```python
from build123d import *

# Parameters (mm, degrees)
BOSS_EXTRUDE2_DEPTH = 503
SHELL1_START        = -463
SHELL1_DEPTH        = 926
FILLET1_R           = 10
SKETCH8_W           = 131.571198008
SKETCH8_H           = 57.2
CUT_EXTRUDE5_DEPTH  = 1006
LPATTERN1_COUNT     = 5
LPATTERN1_PITCH     = 177.2
BOSS_EXTRUDE4_START = -350
SKETCH12_R          = 38
BOSS_EXTRUDE4_DEPTH = 50


# Read off the part's stored shape, not the designer's step: Shell1
with BuildPart() as part:
    # Sketch1 → Boss-Extrude2 (new, symmetric)
    with BuildSketch(Plane.XY):
        with BuildLine():
            ThreePointArc((-150, 150), (-106.066017178, 43.933982822), (0, 0))
            Line((0, 0), (758, 0))
            Line((758, 0), (758, -25))
            Line((758, -25), (777.984855583, -25))
            Line((777.984855583, -25), (794.363516125, 20))
            Line((794.363516125, 20), (356.523002694, 778.362014874))
            Line((356.523002694, 778.362014874), (50.523002694, 778.362014874))
            Line((50.523002694, 778.362014874), (-150, 300))
            Line((-150, 300), (-150, 150))
        make_face()
        Polygon((794.363516125, 20), (777.984855583, -25), (918, -25), align=None)
    extrude(amount=BOSS_EXTRUDE2_DEPTH, both=True)

    # Shell1 outline → Shell1 (cut)
    with BuildSketch(Plane.XY.offset(SHELL1_START)):
        with BuildLine():
            ThreePointArc((-110, 150), (-77.781745931, 72.218254069), (0, 40))
            Line((0, 40), (782.816510741, 40))
            Line((782.816510741, 40), (379.617013461, 738.362014874))
            Line((379.617013461, 738.362014874), (77.127737155, 738.362014874))
            Line((77.127737155, 738.362014874), (-110, 291.955367349))
            Line((-110, 291.955367349), (-110, 150))
        make_face()
    extrude(amount=SHELL1_DEPTH, mode=Mode.SUBTRACT)

    # Fillet1
    fillet1_edges = [part.edges().sort_by_distance(p)[0] for p in [
        (-77.781745931, 72.218254069, 463),
        (391.408255371, 40, -463),
        (-16.436131422, 515.158691112, 463),
        (-110, 220.977683675, 463),
        (391.408255371, 40, 463),
        (-77.781745931, 72.218254069, -463),
        (-110, 220.977683675, -463),
        (-16.436131422, 515.158691112, -463),
    ]]
    fillet(fillet1_edges, radius=FILLET1_R)

    # Sketch8 → Cut-Extrude5 (cut)
    with BuildSketch(Plane(origin=(99.350755487, 272.963957307, 0), x_dir=(0.9396926207859106, -0.3420201433256628, 0), z_dir=(0.34202014332566283, 0.9396926207859106, 0))):
        with Locations((805.402730461, 354.4)):
            Rectangle(SKETCH8_W, SKETCH8_H)
    cut_extrude5 = extrude(amount=-CUT_EXTRUDE5_DEPTH, mode=Mode.SUBTRACT)

    # LPattern1: Cut-Extrude5 ×5
    with Locations(*[(0, 0, i * LPATTERN1_PITCH) for i in range(1, LPATTERN1_COUNT)]):
        add(cut_extrude5, mode=Mode.SUBTRACT)

    # Sketch12 → Boss-Extrude4 (add)
    with BuildSketch(Plane.XY.offset(503).offset(BOSS_EXTRUDE4_START)):
        with BuildLine():
            Line((366.724091876, 760.693210118), (431.275772112, 872.5))
            ThreePointArc((431.275772112, 872.5), (431.275772112, 947.5), (366.323866828, 985))
            Line((366.323866828, 985), (-18.476997306, 985))
            ThreePointArc((-18.476997306, 985), (-71.510005895, 963.033008589), (-93.476997306, 910))
            Line((-93.476997306, 910), (-93.476997306, 434.839679698))
            Line((-93.476997306, 434.839679698), (50.523002694, 778.362014874))
            Line((50.523002694, 778.362014874), (356.523002694, 778.362014874))
            Line((356.523002694, 778.362014874), (366.724091876, 760.693210118))
        make_face()
        with Locations((-18.476997306, 910)):
            Circle(SKETCH12_R, mode=Mode.SUBTRACT)
        with Locations((366.323866828, 910)):
            Circle(SKETCH12_R, mode=Mode.SUBTRACT)
    boss_extrude4 = extrude(amount=BOSS_EXTRUDE4_DEPTH)

    # Mirror2: Boss-Extrude4 across plane
    add(boss_extrude4.mirror(Plane.XY))


solid = part.part
```
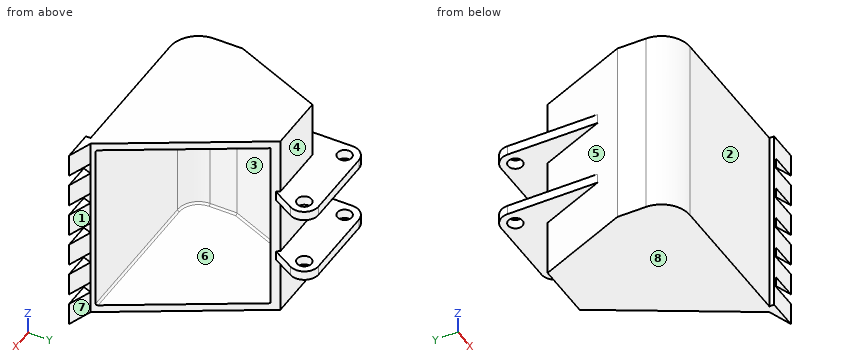
Model file for the job. Use its own axes, mm. Face numbers are marked on the shaded views. A direction names the side the tool comes from. Give positions to 0.01 mm unless a question says otherwise; leave off trailing zeros. Write each loop counter-clockwise with the first axis right and the second up, starting at its lowest first coordinate (ties: lowest second). Pieces come first, ordered by that corner, then holes. Notation, with made-up numbers: (12, 10) -> (18, 10) arc R20 cw to (18, 46) -> close; hole circle Ø3 at (32, -1). An arc over 180 degrees is marked (long way). Use CSV: the item, a comma, the result in double quotes. Start each with the question number.
1) Drill centre lines: L1, parallel to Z at x = 442.5, y = 555; L2, parallel to Y at x = 256, z = 350; L3, parallel to Y at x = 357, z = -198.5. Where is each one in solid material? Low to high.
2) Two-plate mould, pull along Y, no slides. Class the marked faces 6, 7 and 8: released by +Y, released by -Y, zero draft, split by the parting line, or undercut.
3) Cut at A-A on x = 128. List the corners of the cut face in (y, z), plus the area to 3 significant figures.
4) Pin check, flat tips, straight feed: P1, Ø1.5, axis at x = 266, z = -104.5, coming from the +Y side; P2, Ø1, axis at y = 751, z = 374.5, coming from the -X side; P3, Ø5, axis at x = -34.5, z = -109, coming from the -Y side. Stop position of each tip, or through.
5) Cut at B-B on z = 245. List the corners of the cut face in (x, y).
6) Cut at C-C on x = 619. List the corners of the cut face in (y, z), plus the area to 3 significant figures.
7) Tool access for the marked faces 1, 2, 3, 4 and 5: list every direction of +Z, -Z, +X, -X, +Y, -Y with a clear straight run to the whole face (end or side of a thin tool).
Final values:
1,L1,"z = -503 to -463, 463 to 503"
1,L2,"y = 0 to 40, 738.36 to 778.36"
1,L3,"y = 0 to 40, 738.36 to 873.16, 946.84 to 985"
2,face 6,"undercut"
2,face 7,"released by +Y"
2,face 8,"zero draft"
3,outline,"(0, -503) -> (778.36, -503) -> (778.36, -203) -> (985, -203) -> (985, -153) -> (778.36, -153) -> (778.36, 153) -> (985, 153) -> (985, 203) -> (778.36, 203) -> (778.36, 503) -> (0, 503) -> close; hole (40, -453) arc R10 ccw to (50, -463) -> (738.36, -463) -> (738.36, 463) -> (50, 463) arc R10 ccw to (40, 453) -> close"
3,area,"157,000 mm2"
4,P1,"stops at y = 778.36"
4,P2,"stops at x = 38.84"
4,P3,"stops at y = 3.45"
5,outline,"(-150, 150) arc R150 ccw to (0, 0) -> (758, 0) -> (758, -25) -> (918, -25) -> (794.36, 20) -> (782.82, 40) -> (0, 40) arc R110 cw to (-110, 150) -> (-110, 291.96) -> (77.13, 738.36) -> (379.62, 738.36) -> (356.52, 778.36) -> (50.52, 778.36) -> (-150, 300) -> close"
6,outline,"(0, -503) -> (323.74, -503) -> (323.74, -463) -> (50, -463) arc R10 cw to (40, -453) -> (40, 453) arc R10 cw to (50, 463) -> (323.74, 463) -> (323.74, 503) -> (0, 503) -> close"
6,area,"63,000 mm2"
7,face 1,"+Z, -Z, +X, +Y"
7,face 2,"+Z, -Z, -X, -Y"
7,face 3,"+X"
7,face 4,"+Z, +X, -X, +Y"
7,face 5,"-X, +Y"
